from build123d import *

# Parameters (mm, degrees)
EXTRUDE_7_DEPTH = 150
EXTRUDE_START   = 100
EXTRUDE_8_DEPTH = 15


with BuildPart() as part:
    # 草图1 → 凸台-拉伸7 (new body)
    with BuildSketch(Plane.XY):
        with BuildLine():
            Line((0, -15), (0, -18))
            ThreePointArc((0, -18), (5.639478957, -17.09374965), (10.711093494, -14.46625301))
            add(Edge.make_bspline(
                [(10.711093494, -14.46625301), (10.848513024, -13.332455818), (11.044833458, -12.194181271), (11.303579228, -11.074971651), (11.624303017, -10.001858622), (12.335244828, -8.106013793), (12.714420239, -7.26834028), (13.132516135, -6.504930588), (13.58190792, -5.828314757), (14.053066301, -5.245124167)],
                knots=[4.061743838, 4.061743838, 4.061743838, 4.061743838, 4.061743838, 4.061743838, 4.459501644, 4.459501644, 4.459501644, 4.459501644, 4.814431955, 4.814431955, 4.814431955, 4.814431955, 4.814431955, 4.814431955], degree=5, weights=[1, 1, 0.99989411, 0.999870278, 1, 1, 0.999879184, 0.999881196, 1, 1]))
            ThreePointArc((14.053066301, -5.245124167), (14.790408025, -2.498765784), (14.99620502, 0.337394434))
            Line((14.99620502, 0.337394434), (2.680600539, 1.720716673))
            ThreePointArc((2.680600539, 1.720716673), (-1.325193951, 1.356623757), (-4.863483604, -0.556347618))
            Line((-4.863483604, -0.556347618), (-15.368319993, -9.370951957))
            ThreePointArc((-15.368319993, -9.370951957), (-14.001248399, -11.31216351), (-12.390572928, -13.056557835))
            Line((-12.390572928, -13.056557835), (-9.192533317, -7.713451316))
            Line((-9.192533317, -7.713451316), (-9.958577761, -8.356238926))
            Line((-9.958577761, -8.356238926), (-10.408529087, -7.820007816))
            Line((-10.408529087, -7.820007816), (-2.748084656, -1.392131719))
            Line((-2.748084656, -1.392131719), (-2.298133329, -1.928362829))
            Line((-2.298133329, -1.928362829), (-3.064177772, -2.571150439))
            Line((-3.064177772, -2.571150439), (3.624750717, -1.5))
            Line((3.624750717, -1.5), (3.624750717, -3))
            Line((3.624750717, -3), (4.624750717, -3))
            Line((4.624750717, -3), (4.624750717, -2.3))
            Line((4.624750717, -2.3), (6.624750717, -2.3))
            Line((6.624750717, -2.3), (6.624750717, -8.3))
            Line((6.624750717, -8.3), (4.624750717, -8.3))
            Line((4.624750717, -8.3), (4.624750717, -7.6))
            Line((4.624750717, -7.6), (3.624750717, -7.6))
            Line((3.624750717, -7.6), (3.624750717, -8.3))
            Line((3.624750717, -8.3), (4.798277046, -9.121711982))
            Line((4.798277046, -9.121711982), (5.199780551, -8.54830555))
            Line((5.199780551, -8.54830555), (6.83808464, -9.695458423))
            Line((6.83808464, -9.695458423), (3.396626022, -14.610370689))
            Line((3.396626022, -14.610370689), (1.758321933, -13.463217816))
            Line((1.758321933, -13.463217816), (2.159825439, -12.889811385))
            Line((2.159825439, -12.889811385), (1.340673394, -12.316234949))
            Line((1.340673394, -12.316234949), (0, -15))
        make_face()
    extrude_7 = extrude(amount=EXTRUDE_7_DEPTH)

    # 草图5 → 凸台-拉伸8 (add)
    with BuildSketch(Plane.XY.offset(EXTRUDE_START)):
        with BuildLine():
            add(Edge.make_bspline(
                [(7.54460871, -16.342548131), (7.5, -17.169509918), (7.5, -18)],
                knots=[7.753410053, 7.753410053, 7.753410053, 7.853981634, 7.853981634, 7.853981634], degree=2, weights=[0.964895842, 0.981247261, 1]))
            Line((7.5, -18), (10.5, -18))
            add(Edge.make_bspline(
                [(10.711093494, -14.46625301), (10.5, -16.207906554), (10.5, -18)],
                knots=[4.459501644, 4.459501644, 4.459501644, 4.71238898, 4.71238898, 4.71238898], degree=2, weights=[0.920875303, 0.952846219, 1]))
            ThreePointArc((10.711093494, -14.46625301), (9.175935189, -15.485548535), (7.54460871, -16.342548131))
        make_face()
        with BuildLine():
            add(Edge.make_bspline(
                [(7.963401142, -12.711579062), (7.64454263, -14.489960749), (7.54460871, -16.342548131)],
                knots=[7.539833715, 7.539833715, 7.539833715, 7.753410053, 7.753410053, 7.753410053], degree=2, weights=[0.906276709, 0.930171557, 0.964895842]))
            ThreePointArc((7.54460871, -16.342548131), (9.175935189, -15.485548535), (10.711093494, -14.46625301))
            add(Edge.make_bspline(
                [(12, -9), (11.074485981, -11.468037385), (10.711093494, -14.46625301)],
                knots=[4.061743838, 4.061743838, 4.061743838, 4.459501644, 4.459501644, 4.459501644], degree=2, weights=[0.857864376, 0.870589347, 0.920875303]))
            ThreePointArc((12, -9), (10.152748449, -11.041815925), (7.963401142, -12.711579062))
        make_face()
        with BuildLine():
            add(Edge.make_bspline(
                [(17.746791844, -3.00855102), (15.751057332, -3.143384219), (14.053066301, -5.245124167)],
                knots=[3.178841958, 3.178841958, 3.178841958, 3.706813527, 3.706813527, 3.706813527], degree=2, weights=[0.986438278, 0.892660895, 0.865062576]))
            ThreePointArc((17.746791844, -3.00855102), (17.936586258, -1.509593787), (18, 0))
            add(Edge.make_bspline(
                [(18, 0), (16.457794493, 0), (14.980723149, -0.760219655)],
                knots=[6.283185307, 6.283185307, 6.283185307, 6.590751519, 6.590751519, 6.590751519], degree=2, weights=[1, 0.942650708, 0.907759712]))
            ThreePointArc((14.980723149, -0.760219655), (14.689071604, -3.038284946), (14.053066301, -5.245124167))
        make_face()
        with BuildLine():
            ThreePointArc((18, 0), (17.936586258, -1.509593787), (17.746791844, -3.00855102))
            add(Edge.make_bspline(
                [(25.5, -18), (25.5, -3), (18, -3), (17.873359825, -3), (17.746791844, -3.00855102)],
                knots=[1.570796327, 1.570796327, 1.570796327, 3.141592654, 3.141592654, 3.178841958, 3.178841958, 3.178841958], degree=2, weights=[1, 0.707106781, 1, 0.993054435, 0.986438278]))
            Line((25.5, -18), (25.5, -34.982946992))
            Line((25.5, -34.982946992), (28.5, -34.982946992))
            Line((28.5, -34.982946992), (28.5, -18))
            add(Edge.make_bspline(
                [(28.5, -18), (28.5, 0), (18, 0)],
                knots=[4.71238898, 4.71238898, 4.71238898, 6.283185307, 6.283185307, 6.283185307], degree=2, weights=[1, 0.707106781, 1]))
        make_face()
        with BuildLine():
            ThreePointArc((15, 0), (14.995180013, -0.380232008), (14.980723149, -0.760219655))
            add(Edge.make_bspline(
                [(18, 0), (16.457794493, 0), (14.980723149, -0.760219655)],
                knots=[6.283185307, 6.283185307, 6.283185307, 6.590751519, 6.590751519, 6.590751519], degree=2, weights=[1, 0.942650708, 0.907759712]))
            Line((18, 0), (14.99620502, 0.337394434))
            ThreePointArc((14.99620502, 0.337394434), (14.999051225, 0.168707888), (15, 0))
        make_face()
    extrude_8 = extrude(amount=EXTRUDE_8_DEPTH)

    # 镜向1: 凸台-拉伸7, 凸台-拉伸8 across plane
    add(extrude_7.mirror(Plane.XY))
    add(extrude_8.mirror(Plane.XY))


solid = part.part
Model file for the job. Use its own axes, mm. A direction names the side the tool comes from. Give positions to 0.01 mm unless a question says otherwise; leave off trailing zeros. Order: outer loops, then holes, each group sorted by start corner. A loop starts at its lowest first (then second) coordinate and runs counter-clockwise, first axis right, second up. Notation, with made-up numbers: (67.5, 4) - (71.5, 4) arc R6 cw to (71.5, 13) - close; hole circle Ø4 at (-24.75, -34). An arc over 180 degrees is marked (long way). Return JSON: item names as keys, results as strings.
1) Cut at A-A, the plane y = -32. Give the cut face in (x, z).
Geometry says:
{"outline": "(25.5, -115) - (28.5, -115) - (28.5, -100) - (25.5, -100) - close; (25.5, 100) - (28.5, 100) - (28.5, 115) - (25.5, 115) - close"}
2) Flat gauge pins, fed straight in: P1, Ø3.5, axis at x = 9.5, z = -109.5, coming from the -Y side; P2, Ø3, axis at x = 17, z = -31.5, coming from the -Y side; P3, Ø6.5, axis at y = -4, z = -13.5, coming from the -X side; P4, Ø1.6, axis at x = 9.5, y = -16.5, coming from the +Z side. Where does each tip first touch, or does it go through?
Geometry says:
{"P1": "y = -18", "P2": "through", "P3": "x = -12.84", "P4": "z = 115"}
3) 3-axis set-ups, long thin cutter, end or side, ignore diameter. For faces 1 (the flat face through (25.5, -26, 107)), 2 (the flat face through (4, -8, 150)), 3 (the flat face through (-10.04, -4.9, 2.1)), 4 (the flat face through (-10.8, -10.4, 2.1)), 5 (the flat face through (0.233, -2.043, 2.1)): which of +Z, -Z, +X, -X, +Y, -Y reach the whole face in a straight line?
Geometry says:
{"face 1": "+Z, -Z, -X, -Y", "face 2": "+Z, +X, -X, +Y, -Y", "face 3": "+Z, -Z, -X, +Y", "face 4": "+Z, -Z, -Y", "face 5": "+Z, -Z"}
4) Probe line 1 (Y direction, x = 1, z = 25.5); line 2 (X direction, y = -9.5, z = -109); line 3 (Y direction, x = 4, z = -66). List the from-to ranges inside material, lowest first. Write a range as from..to.
Geometry says:
{"line 1": "-17.97..-13, -1.92..1.77", "line 2": "-15.29..-10.26, 6.56..11.82, 24.18..27.26", "line 3": "-17.55..-13.75, -8.56..-7.6, -3..1.57"}
5) Pull direction X, two halves, no side cores. Call faces 6 (the flat face through (25.5, -26, -107)), 7 (the flat face through (4, -8, -150)), 8 (the flat face through (5.14, -12.12, 2.1)): pulls with the +X half, pulls with the -X half, needs draft (parallel to the pull), parting line crosses it, or undercut.
Geometry says:
{"face 6": "pulls with the -X half", "face 7": "needs draft", "face 8": "undercut"}
